The model under review builds one solid part; all positions refer to its coordinate system, in mm. A direction names the side the tool comes from. Round coordinates to 2 decimals unless told otherwise and drop trailing zeros. Order: outer loops, then holes, each group sorted by start corner. A loop starts at its lowest first (then second) coordinate and runs counter-clockwise, first axis right, second up. Notation, with made-up numbers: M 63,87.5 L 118,87.5 A22 cw 118,123.5 Z; hole C -37,70 d5. An arc over 180 degrees is marked long. Answer as a JSON object with one key per item and string values. Group by question number.
1) Insertion check: pin 1 Ø3 at (y, z) = (-27, 16) entering from -X; pin 2 Ø1.5 at (x, y) = (3.5, -4) entering from -Z; pin 3 Ø12 at (y, z) = (-18.5, 10) entering from +X; pin 4 Ø15 at (x, z) = (0, 1) entering from -Y. Each pin has a flat end and moves straight along its axis. Give the tip position at first contact, or say it passes through.
2) Consider section D-D, the plane x = -11.5. Write out the cut boundary in (y, z), then the cut area to 3 significant figures.
3) Consider section A-A, the plane z = 0. Write out the cut boundary in (x, y).
4) Consider section B-B, the plane x = 0. Write out the cut boundary in (y, z), then the cut area to 3 significant figures.
5) To check wall thickness, follow line 1 (Z direction, x = 0, y = -29.15); line 2 (Z direction, x = -0.5, y = -24.25); line 3 (Y direction, x = 13.5, z = 5). State the ranges of each line that lie inside material, in increasing order.
6) Consider section C-C, the plane y = -9. Write out the cut boundary in (x, z).
7) For faces 1 (the cylindrical face through (9.014, -14.05, 2.839)), 2 (the cylindrical face through (9.41, -19.86, -18.1)), list the 3-axis set-ups (+Z, -Z, +X, -X, +Y, -Y) from which the entire face can be reached by the end or side of a thin tool; tool diameter is ignored.
8) The part is to be moulded in two halves that separate along Z. For faces 3 (the cylindrical face through (-14.985, -29.26, 0.66)), 4 (the flat face through (-11, -30, 11)), 5 (the cylindrical face through (23.846, -4.93, 7.509)), say which applies: +Z half, -Z half, draft (parallel to the pull), parting line (faces both ways), or undercut.
```python
from build123d import *

# Parameters (mm, degrees)
F0_R     = 20.4
F0_R_2   = 9.45
F1_DEPTH = 30
F0_R_3   = 25
F2_DEPTH = 10
F3_R     = 15
F3_R_2   = 9.45
F4_DEPTH = 1.5


with BuildPart() as f1:
    # F0 (on Front) → F1 (new body)
    with BuildSketch(Plane.XZ):
        Circle(F0_R)
        Circle(F0_R_2, mode=Mode.SUBTRACT)
    extrude(amount=F1_DEPTH)

    # F0 (on Front) → F2 (join)
    with BuildSketch(Plane.XZ):
        Circle(F0_R_3)
        Circle(F0_R, mode=Mode.SUBTRACT)
    extrude(amount=F2_DEPTH)

    # F3 (on face) → F4 (cut)
    with BuildSketch(Plane.XZ.offset(30)):
        Circle(F3_R)
        Circle(F3_R_2, mode=Mode.SUBTRACT)
    extrude(amount=-F4_DEPTH, mode=Mode.SUBTRACT)


solid = f1.part
```
Results list:
{
 "1": {"pin 1": "x = -14.35", "pin 2": "z = -24.85", "pin 3": "x = 20", "pin 4": "through"},
 "2": {"outline": "M -30,-16.85 L -10,-16.85 L -10,-22.2 L 0,-22.2 L 0,22.2 L -10,22.2 L -10,16.85 L -30,16.85 L -30,9.63 L -28.5,9.63 L -28.5,-9.63 L -30,-9.63 Z", "area": "1,090 mm^2"},
 "3": {"outline": "M -25,-10 L -20.4,-10 L -20.4,-30 L -15,-30 L -15,-28.5 L -9.45,-28.5 L -9.45,0 L -25,0 Z; M 9.45,-28.5 L 15,-28.5 L 15,-30 L 20.4,-30 L 20.4,-10 L 25,-10 L 25,0 L 9.45,0 Z"},
 "4": {"outline": "M -30,-20.4 L -10,-20.4 L -10,-25 L 0,-25 L 0,-9.45 L -28.5,-9.45 L -28.5,-15 L -30,-15 Z; M -30,15 L -28.5,15 L -28.5,9.45 L 0,9.45 L 0,25 L -10,25 L -10,20.4 L -30,20.4 Z", "area": "732 mm^2"},
 "5": {"line 1": "-20.4 to -15, 15 to 20.4", "line 2": "-20.39 to -9.44, 9.44 to 20.39", "line 3": "-28.5 to 0"},
 "6": {"outline": "C 0,0 d50; hole C 0,0 d18.9"},
 "7": {"face 1": "+Y, -Y", "face 2": "-Y"},
 "8": {"face 3": "undercut", "face 4": "draft", "face 5": "parting line"}
}
